For this review, take the finished solid that the model builds, in its own axes (mm). Round coordinates to 2 decimals unless told otherwise and drop trailing zeros. Write each loop counter-clockwise with the first axis right and the second up, starting at its lowest first coordinate (ties: lowest second). Pieces come first, ordered by that corner, then holes. Notation, with made-up numbers: (1, 48.5) - (19, 48.5) arc R33 ccw to (19, 76.5) - close; hole circle Ø11 at (40, 50.5). An arc over 180 degrees is marked (long way). Answer in a Markdown table with one row per item. Add a question column.
from build123d import *

# Parameters (mm, degrees)
SKETCH004_W             = 50
SKETCH004_H             = 50
PAD002_DEPTH            = 4
SKETCH005_W             = 26
SKETCH005_H             = 26
POCKET_DEPTH            = 10
SKETCH006_R             = 1.5
HOLE002_DEPTH           = 5
POLARPATTERN001_COUNT   = 4
SKETCH007_W             = 5.6
SKETCH007_H             = 5.6
POCKET001_DEPTH         = 2
POLARPATTERN002_COUNT   = 4
FILLET013_R             = 1
FILLET014_R             = 1
BODY001_PLACEMENT_ANGLE = 180


with BuildPart() as part:
    # Sketch004 → Pad002 (new body)
    with BuildSketch(Plane.XY):
        Rectangle(SKETCH004_W, SKETCH004_H)
    extrude(amount=PAD002_DEPTH)

    # Sketch005 (on Face6 of Pad002) → Pocket (cut)
    with BuildSketch(Plane.XY.offset(4)):
        Rectangle(SKETCH005_W, SKETCH005_H)
    extrude(amount=-POCKET_DEPTH, mode=Mode.SUBTRACT)

    # Sketch006 (on Face5 of Pocket) → Hole002 (cut)
    with BuildSketch(Plane.XY.offset(4)):
        with Locations((-18.636039, 18.636039)):
            Circle(SKETCH006_R)
    hole002 = extrude(amount=-HOLE002_DEPTH, mode=Mode.SUBTRACT)

    # PolarPattern001: Hole002 ×4 about axis
    polarpattern001_axis = Axis((0, 0, 4), (0, 0, 1))
    for i in range(1, POLARPATTERN001_COUNT):
        add(hole002.rotate(polarpattern001_axis, i * 360 / POLARPATTERN001_COUNT), mode=Mode.SUBTRACT)

    # Sketch007 (on Face4 of PolarPattern001) → Pocket001 (cut)
    with BuildSketch(Plane(origin=(0, 0, 0), x_dir=(1, 0, 0), z_dir=(0, 0, -1))):
        with Locations((-18.636039, 18.636039)):
            Rectangle(SKETCH007_W, SKETCH007_H)
    pocket001 = extrude(amount=-POCKET001_DEPTH, mode=Mode.SUBTRACT)

    # PolarPattern002: Pocket001 ×4 about axis
    polarpattern002_axis = Axis((0, 0, 0), (0, 0, -1))
    for i in range(1, POLARPATTERN002_COUNT):
        add(pocket001.rotate(polarpattern002_axis, i * 360 / POLARPATTERN002_COUNT), mode=Mode.SUBTRACT)

    # Fillet013
    fillet013_edges = [part.edges().sort_by_distance(p)[0] for p in [
        (-25, 0, 0),
        (0, -25, 0),
        (0, 25, 0),
        (25, 0, 0),
        (-18.636039, -21.436039, 0),
        (-15.836039, -18.636039, 0),
        (-21.436039, -18.636039, 0),
        (-18.636039, -15.836039, 0),
        (21.436039, -18.636039, 0),
        (18.636039, -15.836039, 0),
        (15.836039, -18.636039, 0),
        (18.636039, -21.436039, 0),
        (0, -13, 0),
        (13, 0, 0),
        (-13, 0, 0),
        (0, 13, 0),
        (-21.436039, 18.636039, 0),
        (-18.636039, 15.836039, 0),
        (-15.836039, 18.636039, 0),
        (-18.636039, 21.436039, 0),
        (18.636039, 21.436039, 0),
        (15.836039, 18.636039, 0),
        (18.636039, 15.836039, 0),
        (21.436039, 18.636039, 0),
    ]]
    fillet(fillet013_edges, radius=FILLET013_R)

    # Fillet014
    fillet014_edges = [part.edges().sort_by_distance(p)[0] for p in [
        (-25, 0, 4),
        (0, -25, 4),
        (0, 25, 4),
        (25, 0, 4),
        (-18.636039, -20.136039, 4),
        (20.136039, -18.636039, 4),
        (-20.136039, 18.636039, 4),
        (0, -13, 4),
        (13, 0, 4),
        (-13, 0, 4),
        (0, 13, 4),
        (18.636039, 20.136039, 4),
    ]]
    fillet(fillet014_edges, radius=FILLET014_R)


with BuildPart() as part_1:
    # Body001 placement: moved
    add(part.part.moved(Location((0, 0, 12))).rotate(Axis((0, 0, 12), (1, 0, 0)), BODY001_PLACEMENT_ANGLE))


solid = part_1.part
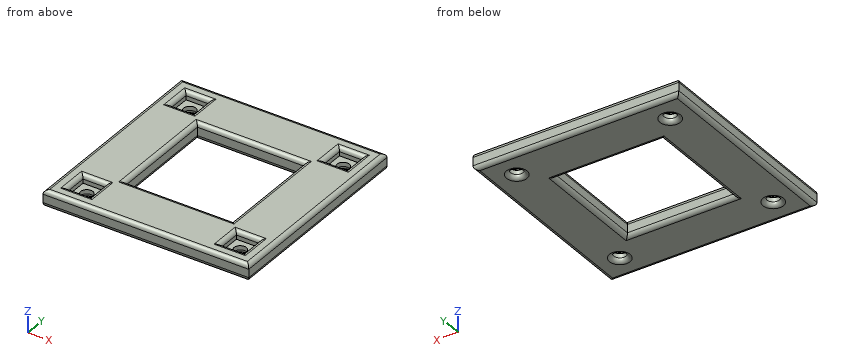
Q1. Insertion check: pin 1 Ø2 at (x, y) = (12.5, -10) entering from -Z; pin 2 Ø2.5 at (x, y) = (-18.64, -18.64) entering from -Z; pin 3 Ø5 at (x, y) = (18.64, 18.64) entering from -Z; pin 4 Ø4.5 at (x, y) = (-19.5, -18.5) entering from +Z. Each pin has a flat end and moves straight along its axis. Give the tip position at first contact, or say it passes through.
Q2. To check wall thickness, follow probe 1 along Y at (x, z) = (-18.5, 10.3); probe 2 along X at (y, z) = (12, 10.2). State the ranges of each line that lie inside material, in increasing order.
Q3. Add section A-A on x = -8.5. State the section outline as (y, z) points.
Q4. Add section C-C on x = 18. Count the separate pieces of the cut face and the enclosed holes in it, then the cut area to 3 significant figures.
Answer sheet:
| question | item | result |
|---|---|---|
| 1 | pin 1 | stops at z = 8.13 |
| 1 | pin 2 | passes through |
| 1 | pin 3 | stops at z = 8 |
| 1 | pin 4 | stops at z = 11.73 |
| 2 | probe 1 | y = -25 to -21.44, -15.84 to 15.84, 21.44 to 25 |
| 2 | probe 2 | x = -25 to -13, 13 to 25 |
| 3 | outline | (-25, 9) arc R1 ccw to (-24, 8) - (-14, 8) arc R1 ccw to (-13, 9) - (-13, 11) arc R1 ccw to (-14, 12) - (-24, 12) arc R1 ccw to (-25, 11) - close; (13, 9) arc R1 ccw to (14, 8) - (24, 8) arc R1 ccw to (25, 9) - (25, 11) arc R1 ccw to (24, 12) - (14, 12) arc R1 ccw to (13, 11) - close |
| 4 | separate pieces | 3 |
| 4 | enclosed holes | 0 |
| 4 | area | 164 mm² |
